Read the model definition and answer for the solid it produces. Units are mm, in the model's axes. A direction names the side the tool comes from. Give positions to 0.01 mm unless a question says otherwise; leave off trailing zeros. Loops run counter-clockwise (first coordinate to the right, second up) from the corner with the lowest first, then second, coordinate; pieces in that order, holes last. Notation, with made-up numbers: M 61,-31 L 87,-31 A33 cw 87,6 Z; hole C 32,-23.5 d5. An arc over 180 degrees is marked long. Return JSON: item names as keys, results as strings. Group by question number.
```python
from build123d import *

# Parameters (mm, degrees)
BOSS_EXTRUDE1_DEPTH = 3.2
SKETCH3_R           = 12.3
BOSS_EXTRUDE2_DEPTH = 3.2
SKETCH4_R           = 4
BOSS_EXTRUDE3_DEPTH = 4
SKETCH6_W           = 3.2
SKETCH6_H           = 65
BOSS_EXTRUDE4_DEPTH = 190
SKETCH8_W           = 3.2
SKETCH8_H           = 89
BOSS_EXTRUDE5_DEPTH = 190
SKETCH9_W           = 194.2
SKETCH9_H           = 190
BOSS_EXTRUDE7_DEPTH = 3.2
SKETCH11_R          = 6.2
CUT_EXTRUDE2_DEPTH  = 94
SKETCH12_R          = 35
BOSS_EXTRUDE8_DEPTH = 20
SKETCH14_W          = 90
SKETCH14_H          = 85
BOSS_EXTRUDE9_DEPTH = 80
SKETCH15_W          = 80
SKETCH15_H          = 78
CUT_EXTRUDE3_DEPTH  = 88
SKETCH16_W          = 83.876304214
SKETCH16_H          = 71.530824042
CUT_EXTRUDE7_DEPTH  = 10


with BuildPart() as part:
    # Sketch1 → Boss-Extrude1 (new body)
    with BuildSketch(Plane(origin=(0, 0, 0), x_dir=(1, 0, 0), z_dir=(0, 1, 0))):
        Polygon((-71.199297972, 0), (119.800702028, 0), (119.800702028, -90), (46.272924854, -150.155348756), (-15.035731115, -153.181069815), (-74.399297972, -109), (-74.399297972, -65), (-71.199297972, -65), align=None)
    boss_extrude1 = extrude(amount=BOSS_EXTRUDE1_DEPTH)

    # Sketch3 → Boss-Extrude2 (add)
    with BuildSketch(Plane.XZ):
        with Locations(Location((-5.399297972, 108.199281837, 0), (0, 0, 270))):
            Circle(SKETCH3_R)
    boss_extrude2 = extrude(amount=BOSS_EXTRUDE2_DEPTH)

    # Sketch4 → Boss-Extrude3 (add)
    with BuildSketch(Plane.XZ.offset(3.2)):
        with Locations(Location((-5.399297972, 108.199281837, 0), (0, 0, 270))):
            Circle(SKETCH4_R)
    boss_extrude3 = extrude(amount=BOSS_EXTRUDE3_DEPTH)

    # Sketch6 → Boss-Extrude4 (add)
    with BuildSketch(Plane(origin=(0, 0, 0), x_dir=(1, 0, 0), z_dir=(0, 1, 0))):
        with Locations((-72.799297972, -32.5)):
            Rectangle(SKETCH6_W, SKETCH6_H)
    extrude(amount=BOSS_EXTRUDE4_DEPTH)

    # Sketch8 → Boss-Extrude5 (add)
    with BuildSketch(Plane(origin=(0, 0, 0), x_dir=(1, 0, 0), z_dir=(0, 1, 0))):
        with Locations((118.200702028, -44.5)):
            Rectangle(SKETCH8_W, SKETCH8_H)
    extrude(amount=BOSS_EXTRUDE5_DEPTH)

    # Mirror1: Boss-Extrude1, Boss-Extrude2, Boss-Extrude3 across plane
    add(boss_extrude1.mirror(Plane(origin=(0, 95, 0), x_dir=(0, 0, 1), z_dir=(0, -1, 0))))
    add(boss_extrude2.mirror(Plane(origin=(0, 95, 0), x_dir=(0, 0, 1), z_dir=(0, -1, 0))))
    add(boss_extrude3.mirror(Plane(origin=(0, 95, 0), x_dir=(0, 0, 1), z_dir=(0, -1, 0))))

    # Sketch9 → Boss-Extrude7 (add)
    with BuildSketch(Plane.XY):
        with Locations((22.700702028, 95)):
            Rectangle(SKETCH9_W, SKETCH9_H)
    extrude(amount=-BOSS_EXTRUDE7_DEPTH)

    # Sketch11 → Cut-Extrude2 (cut, symmetric)
    with BuildSketch(Plane(origin=(0, 95, 0), x_dir=(1, 0, 0), z_dir=(0, 1, 0))):
        with Locations(Location((-5.399297972, -108.199281837, 0), (0, 0, 270))):
            Circle(SKETCH11_R)
    extrude(amount=CUT_EXTRUDE2_DEPTH, both=True, mode=Mode.SUBTRACT)

    # Sketch12 → Boss-Extrude8 (add)
    with BuildSketch(Plane(origin=(0, 0, -3.2), x_dir=(-1, 0, 0), z_dir=(0, 0, -1))):
        with Locations((-22.700702028, 95)):
            Circle(SKETCH12_R)
    extrude(amount=BOSS_EXTRUDE8_DEPTH)

    # Sketch14 → Boss-Extrude9 (add)
    with BuildSketch(Plane(origin=(0, 190, 0), x_dir=(1, 0, 0), z_dir=(0, 1, 0))):
        with Locations((13.00356987, -98.058145234)):
            Rectangle(SKETCH14_W, SKETCH14_H)
    extrude(amount=BOSS_EXTRUDE9_DEPTH)

    # Sketch15 → Cut-Extrude3 (cut)
    with BuildSketch(Plane(origin=(58.00356987, 0, 0), x_dir=(0, 0, -1), z_dir=(1, 0, 0))):
        with Locations((-98.058145234, 230)):
            Rectangle(SKETCH15_W, SKETCH15_H)
    extrude(amount=-CUT_EXTRUDE3_DEPTH, mode=Mode.SUBTRACT)

    # Sketch16 → Cut-Extrude7 (cut)
    with BuildSketch(Plane.XY.offset(58.058145234)):
        with Locations((13.00356987, 230)):
            Rectangle(SKETCH16_W, SKETCH16_H)
    extrude(amount=-CUT_EXTRUDE7_DEPTH, mode=Mode.SUBTRACT)


solid = part.part
```
1. Find section B-B (y = 95). Write down the section's boundary in (x, z).
2. Straight lines are drawn through the part: line 1 along Y through (x, z) = (32, 68); line 2 along Y through (x, z) = (-48, 96); line 3 along X through (y, z) = (42, 35). For each, find the intervals that lie inside material, in ascending order.
3. Flat-ended cylindrical pins translate along their axes: P1, Ø6, axis at y = 221.5, z = 56, coming from the +X side; P2, Ø2, axis at y = 234.5, z = 74, coming from the -X side; P3, Ø1, axis at x = -73, y = 74.5, coming from the +Z side. Find the tip coordinate at first contact, or state that the pin passes through.
4. The mould has two halves that part along Y. Classify faces 1 (the flat face through (15, 269, 99)), 2 (the cylindrical face through (-6.931, -5.172, 104.504)), 3 (the cylindrical face through (27.26, 129.7, -13.06)): +Y half, -Y half, draft (parallel to the pull), parting line (faces both ways), or undercut.
5. Find section C-C (x = -41). Write down the section's boundary in (y, z).
6. Find section D-D (z = 77). Write down the section's boundary in (x, y), and give its area (3 significant figures).
7. For faces 4 (the cylindrical face through (-5.127, 187.915, 102.005)), 5 (the cylindrical face through (-4.858, -1.578, 120.487)), 6 (the flat face through (116.601, 94, 45)), determine the directions among +Z, -Z, +X, -X, +Y, -Y from which every point of the face is accessible in a straight line to the end or side of a thin tool.
8. Find section A-A (z = 43). Write down the section's boundary in (x, y), and give its area (3 significant figures).
Result:
{
 "1": {"outline": "M -74.4,-3.2 L -12.3,-3.2 L -12.3,-23.2 L 57.7,-23.2 L 57.7,-3.2 L 119.8,-3.2 L 119.8,89 L 116.6,89 L 116.6,0 L -71.2,0 L -71.2,65 L -74.4,65 Z"},
 "2": {"line 1": "y = 0 to 3.2, 186.8 to 191, 269 to 270", "line 2": "y = 0 to 3.2, 186.8 to 190", "line 3": "x = -74.4 to -71.2, 116.6 to 119.8"},
 "3": {"P1": "stops at x = 58", "P2": "stops at x = -32", "P3": "stops at z = 65"},
 "4": {"face 1": "undercut", "face 2": "draft", "face 3": "parting line"},
 "5": {"outline": "M 0,-3.2 L 190,-3.2 L 190,133.86 L 186.8,133.86 L 186.8,0 L 3.2,0 L 3.2,133.86 L 0,133.86 Z"},
 "6": {"outline": "M -74.4,0 L 119.8,0 L 119.8,190 L 58,190 L 58,191 L -30,191 L -30,269 L 58,269 L 58,270 L -32,270 L -32,190 L -74.4,190 L -74.4,186.8 L 116.6,186.8 L 116.6,3.2 L -74.4,3.2 Z", "area": "2,170 mm2"},
 "7": {"face 4": "none", "face 5": "-Y", "face 6": "+Z"},
 "8": {"outline": "M -74.4,0 L 119.8,0 L 119.8,190 L -74.4,190 Z; hole M -71.2,3.2 L 116.6,3.2 L 116.6,186.8 L -71.2,186.8 Z", "area": "2,420 mm2"}
}
